Input: part model. Units: mm. Frame: model coordinates. Face numbers are marked on the shaded views. A direction names the side the tool comes from. Round coordinates to 2 decimals unless told otherwise and drop trailing zeros. Loops run counter-clockwise (first coordinate to the right, second up) from the corner with the lowest first, then second, coordinate; pieces in that order, holes last. Notation, with made-up numbers: (14, 20) -> (46, 20) arc R15 cw to (46, 27) -> close; hole circle Ø5 at (88, 60.25). An arc over 180 degrees is marked (long way). Answer in a Markdown table with one row per item. Add a question column.
Q1. Mould query, pull axis Y, two halves, no side actions, for the marked faces 4, 5 and 6. Classes: pulls with the +Y half, pulls with the -Y half, needs draft (parallel to the pull), parting line crosses it, or undercut.
Q2. Ray query, L1, parallel to X at y = 0.75, z = 9; L2, parallel to X at y = -0.25, z = 5.25; L3, parallel to Z at x = 14.5, y = -1.75. Return the intervals inside material, ascending. Write a range as from..to.
Q3. Section A-A, the plane y = 7.5. Output: boundary loops of the cut face in (x, z), and give its area (3 significant figures).
Q4. Reachability of the marked faces 1, 2 and 3 from +Z, -Z, +X, -X, +Y, -Y: full face, straight path, thin tool, end or side. Return the list, or none.
Q5. Section B-B, the plane y = 5.5. Output: boundary loops of the cut face in (x, z), and give its area (3 significant figures).
Q6. Pin query (flat end, axial travel): pin 1 (3.5 mm diameter, centred on y = 2.5, z = 6, fed in from +X); pin 2 (5.5 mm diameter, centred on y = 4, z = 5, fed in from -X); pin 3 (3 mm diameter, centred on y = -1.5, z = 4.5, fed in from -X). Return the tip coordinate at first contact, or that it passes through.
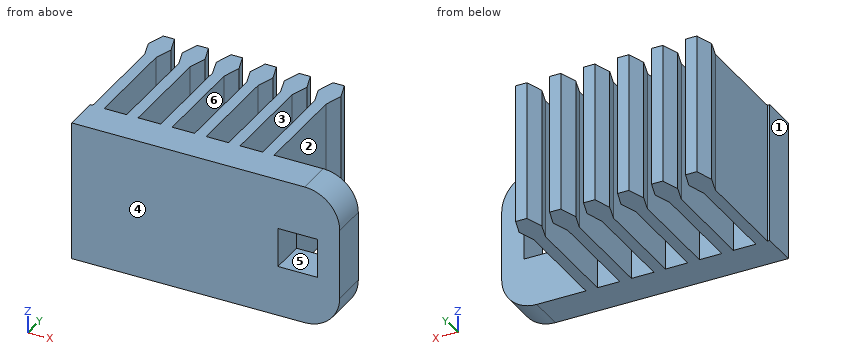
```python
from build123d import *

# Parameters (mm, degrees)
RESSALTO_EXTRUS_O1_DEPTH = 10
ESBO_O2_W                = 2.8
ESBO_O2_H                = 2.8
CORTE_EXTRUS_O1_DEPTH    = 24.091998614


with BuildPart() as part:
    # Esboço1 → Ressalto-extrusão1 (new body)
    with BuildSketch(Plane.XY):
        Polygon((-0.4, 7), (-0.4, 0), (-0.57, 0), (-0.57, -2.5), (5.43, -2.5), (18.52, -2.5), (18.52, 0), (12.52, 0), (12.52, 7), (12.92, 8.25), (12.5, 9.5), (11.7, 9.5), (11.3, 8.25), (11.7, 7), (11.7, 0), (10.1, 0), (10.1, 7), (10.5, 8.25), (10.08, 9.5), (9.28, 9.5), (8.88, 8.25), (9.28, 7), (9.28, 0), (7.68, 0), (7.68, 7), (8.08, 8.25), (7.66, 9.5), (6.86, 9.5), (6.46, 8.25), (6.86, 7), (6.86, 0), (5.26, 0), (5.26, 7), (5.66, 8.25), (5.24, 9.5), (4.44, 9.5), (4.04, 8.25), (4.44, 7), (4.44, 0), (2.84, 0), (2.84, 7), (3.24, 8.25), (2.82, 9.5), (2.02, 9.5), (1.62, 8.25), (2.02, 7), (2.02, 0), (0.42, 0), (0.42, 7), (0.82, 8.25), (0.4, 9.5), (-0.4, 9.5), (-0.8, 8.25), align=None)
    extrude(amount=RESSALTO_EXTRUS_O1_DEPTH)

    # Esboço2 → Corte-extrusão1 (cut, through all)
    with BuildSketch(Plane(origin=(0, 0, 0), x_dir=(1, 0, 0), z_dir=(0, 1, 0))):
        with Locations((15.52, -5)):
            Rectangle(ESBO_O2_W, ESBO_O2_H)
        with BuildLine():
            ThreePointArc((16.02, 0), (17.787766953, -0.732233047), (18.52, -2.5))
            Line((18.52, -2.5), (18.52, 0))
            Line((18.52, 0), (16.02, 0))
        make_face()
        with BuildLine():
            Line((18.52, -10), (18.52, -7.5))
            ThreePointArc((18.52, -7.5), (17.787766953, -9.267766953), (16.02, -10))
            Line((16.02, -10), (18.52, -10))
        make_face()
    extrude(amount=-CORTE_EXTRUS_O1_DEPTH, mode=Mode.SUBTRACT)


solid = part.part
```
Answer block:
| question | item | result |
|---|---|---|
| 1 | face 4 | pulls with the -Y half |
| 1 | face 5 | needs draft |
| 1 | face 6 | undercut |
| 2 | L1 | -0.4..0.42, 2.02..2.84, 4.44..5.26, 6.86..7.68, 9.28..10.1, 11.7..12.52 |
| 2 | L2 | -0.57..14.12, 16.92..18.52 |
| 2 | L3 | 0..3.6, 6.4..10 |
| 3 | outline | (-0.56, 0) -> (0.58, 0) -> (0.58, 10) -> (-0.56, 10) -> close; (1.86, 0) -> (3, 0) -> (3, 10) -> (1.86, 10) -> close; (4.28, 0) -> (5.42, 0) -> (5.42, 10) -> (4.28, 10) -> close; (6.7, 0) -> (7.84, 0) -> (7.84, 10) -> (6.7, 10) -> close; (9.12, 0) -> (10.26, 0) -> (10.26, 10) -> (9.12, 10) -> close; (11.54, 0) -> (12.68, 0) -> (12.68, 10) -> (11.54, 10) -> close |
| 3 | area | 68.4 mm^2 |
| 4 | face 1 | +Z, -Z, -X, -Y |
| 4 | face 2 | +Z, -Z, +X |
| 4 | face 3 | +Z, -Z |
| 5 | outline | (-0.4, 0) -> (0.42, 0) -> (0.42, 10) -> (-0.4, 10) -> close; (2.02, 0) -> (2.84, 0) -> (2.84, 10) -> (2.02, 10) -> close; (4.44, 0) -> (5.26, 0) -> (5.26, 10) -> (4.44, 10) -> close; (6.86, 0) -> (7.68, 0) -> (7.68, 10) -> (6.86, 10) -> close; (9.28, 0) -> (10.1, 0) -> (10.1, 10) -> (9.28, 10) -> close; (11.7, 0) -> (12.52, 0) -> (12.52, 10) -> (11.7, 10) -> close |
| 5 | area | 49.2 mm^2 |
| 6 | pin 1 | x = 12.52 |
| 6 | pin 2 | x = -0.4 |
| 6 | pin 3 | x = -0.57 |
